Drawing for the job (mm, zero at the part's lowest x, y, z). A direction names the side the tool comes from. Coordinates: 2 decimals unless noted, no trailing zeros. Write each loop counter-clockwise with the first axis right and the second up, starting at its lowest first coordinate (ties: lowest second). Pieces come first, ordered by that corner, then holes. Notation, with made-up numbers: (5, 84) -> (33, 84) arc R9 ccw to (33, 90) -> close; hole circle Ø8 at (46, 61.5). An arc over 180 degrees is marked (long way). Answer as CSV lines item,"result".
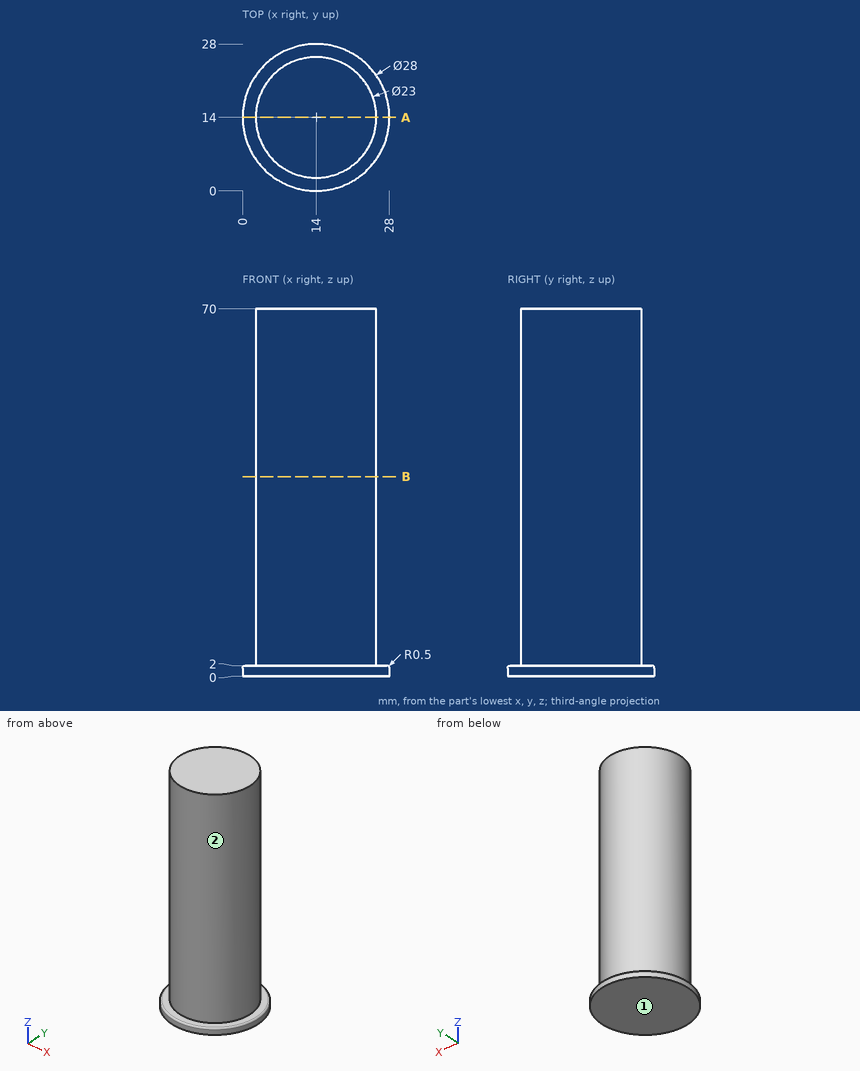
Item 1: Saw through at A-A on y = 14. Give the cut face in (x, z).
Answer below:
outline,"(0, 0) -> (28, 0) -> (28, 1.5) arc R0.5 ccw to (27.5, 2) -> (25.5, 2) -> (25.5, 70) -> (2.5, 70) -> (2.5, 2) -> (0.5, 2) arc R0.5 ccw to (0, 1.5) -> close"
Item 2: Wall check: line 1 (Z direction, x = 4.5, y = 4.75); line 2 (Y direction, x = 4.75, z = 14); line 3 (Y direction, x = 11.25, z = 40). Give the ranges that are in metal, low to high. Write a range as from..to.
Answer below:
line 1,"z = 0..2"
line 2,"y = 7.17..20.83"
line 3,"y = 2.83..25.17"
Item 3: Flat gauge pins, fed straight in: pin 1 (1.5 mm diameter, centred on x = 18.5, y = 7.5, fed in from -Z); pin 2 (3 mm diameter, centred on x = 16, z = 39, fed in from -Y); pin 3 (10 mm diameter, centred on y = 14.5, z = 45.5, fed in from -X); pin 4 (2 mm diameter, centred on y = 24.5, z = 61, fed in from +X). Where does each tip first touch, or does it go through?
Answer below:
pin 1,"stops at z = 0"
pin 2,"stops at y = 2.51"
pin 3,"stops at x = 2.5"
pin 4,"stops at x = 20.48"
Item 4: 3-axis set-ups, long thin cutter, end or side, ignore diameter. For the marked faces 1 and 2: which of +Z, -Z, +X, -X, +Y, -Y reach the whole face in a straight line?
Answer below:
face 1,"-Z, +X, -X, +Y, -Y"
face 2,"+Z"
Item 5: Saw through at B-B on z = 38. Give the cut face in (x, y), and give its area (3 significant figures).
Answer below:
outline,"circle Ø23 at (14, 14)"
area,"415 mm2"
